Source: CAD feature listing. Evaluate the final solid. Frame: model axes, mm. Coordinates: 2 decimals unless noted, no trailing zeros. Order: outer loops, then holes, each group sorted by start corner. A loop starts at its lowest first (then second) coordinate and runs counter-clockwise, first axis right, second up. Notation, with made-up numbers: (22, -4) - (54, -4) arc R3 cw to (54, 0) - close; hole circle Ø6 at (21, 74). An arc over 180 degrees is marked (long way). One line per question, with ' | ' between items.
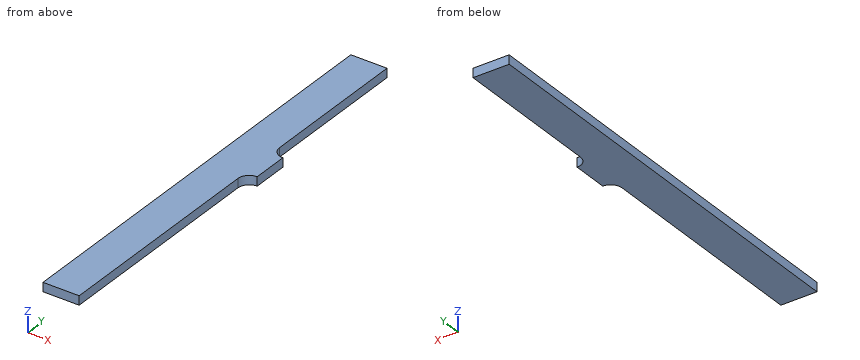
Autodesk Inventor part; units mm, degrees
ref_plane "YZ Plane" through (0, 0, 0) normal (1, 0, 0) x (0, 1, 0)
ref_plane "XZ Plane" through (0, 0, 0) normal (0, 1, 0) x (-1, 0, 0)
ref_plane "XY Plane" through (0, 0, 0) normal (0, 0, 1) x (1, 0, 0)
sketch "Sketch1" plane through (0, 0, 0) normal (0, 0, 1) x (1, 0, 0)
  line L0 (-4.0353, 2.9403) -> (8.6647, 2.9403)
  line L1 (8.6647, 2.9403) -> (8.6647, -50.241)
  line L2 (8.6647, -149.4597) -> (-4.0353, -149.4597)
  line L3 (-4.0353, -149.4597) -> (-4.0353, 2.9403)
  line L4 (12.6335, -54.2097) -> (12.6335, -54.2097)
  line L5 (12.6335, -54.2097) -> (12.6335, -66.9097)
  line L6 (12.6335, -66.9097) -> (12.6335, -66.9097)
  line L7 (8.6647, -70.8785) -> (8.6647, -149.4597)
  arc A0 (8.6647, -50.241) -> (12.6335, -54.2097) centre (12.6335, -50.241) ccw
  arc A1 (12.6335, -66.9097) -> (8.6647, -70.8785) centre (12.6335, -70.8785) ccw
  point P0 (0, 0)
  point P1 (8.6647, -66.9097)
  dimension "d0" = 12.7
  dimension "d1" = 152.4
  dimension "d2" = 3.9688
  dimension "d3" = 12.7
  dimension "d4" = 3.9688
  dimension "d5" = 57.15
extrude "Extrusion1" add sketch "Sketch1" along normal blind 3.175
properties part number "Granny Gearbox Routing Template Vertical Tabs"
(1) Material intervals for L1, parallel to X at y = -135.5, z = 2.05; L2, parallel to Y at x = 9.5, z = 1.2; L3, parallel to Y at x = 10.75, z = 1.05, sorted ascending. Write a range as from..to.
Taken from the geometry:
L1: x = -4.04..8.66 | L2: y = -68.44..-52.68 | L3: y = -67.39..-53.73
(2) Cut plane B-B (y = -92.5). Return the cut outline in (x, z) (3 decimals), and give its area (3 significant figures).
Taken from the geometry:
outline: (-4.035, 0) - (8.665, 0) - (8.665, 3.175) - (-4.035, 3.175) - close | area: 40.3 mm²
(3) Pin query (flat end, axial travel): P1, Ø1, axis at y = -94.5, z = 1.5, coming from the +X side. Return the tip coordinate at first contact, or that it passes through.
Taken from the geometry:
P1: stops at x = 8.66
(4) Cut plane A-A (z = 0.7). Return the cut outline in (x, y), and give its area (3 significant figures).
Taken from the geometry:
outline: (-4.04, -149.46) - (8.66, -149.46) - (8.66, -70.88) arc R3.97 cw to (12.63, -66.91) - (12.63, -54.21) arc R3.97 cw to (8.66, -50.24) - (8.66, 2.94) - (-4.04, 2.94) - close | area: 1,990 mm²
